Autodesk Fusion 360 part; units mm, degrees
sketch "Sketch1" plane through (0, 0, 0) normal (0, 0, 1) x (1, 0, 0)
  line L0 (4.25, 2.75) -> (-4.25, 2.75)
  line L1 (-4.25, 2.75) -> (-4.25, -2.75)
  line L2 (-4.25, -2.75) -> (4.25, -2.75)
  line L3 (4.25, -2.75) -> (4.25, 2.75)
  line L4 (4.25, 2.75) -> (-4.25, -2.75) construction
  line L5 (-4.25, 2.75) -> (4.25, -2.75) construction
  line L6 (-6.25, -4.75) -> (6.25, -4.75)
  line L7 (6.25, -4.75) -> (6.25, 4.75)
  line L8 (6.25, 4.75) -> (-6.25, 4.75)
  line L9 (-6.25, 4.75) -> (-6.25, -4.75)
  line L10 (-4.25, 2.75) -> (-6.25, 2.75)
  line L11 (4.25, 2.75) -> (6.25, 2.75)
  dimension "d1" = 8.5
  dimension "d2" = 5.5
  dimension "d3" = 2
extrude "Extrude1" add sketch "Sketch1" along normal blind 8.2 contours L1 L2 L3 L6 L7 L9 L10 L11
sketch "Sketch2" plane through (0, 0, 8.2) normal (0, 0, 1) x (-1, 0, 0)
  line L0 (4.25, -2.75) -> (6.25, -2.75)
  line L1 (6.25, -2.75) -> (6.25, 4.75)
  line L2 (6.25, 4.75) -> (-6.25, 4.75)
  line L3 (-6.25, 4.75) -> (-6.25, -2.75)
  line L4 (-6.25, -2.75) -> (-4.25, -2.75)
  line L5 (-4.25, -2.75) -> (-4.25, 2.75)
  line L6 (-4.25, 2.75) -> (4.25, 2.75)
  line L7 (4.25, 2.75) -> (4.25, -2.75)
  line L8 (6.25, -2.75) -> (-6.25, -2.75)
  line L9 (-6.25, -2.75) -> (-6.25, 4.75)
  line L10 (-6.25, 4.75) -> (6.25, 4.75)
  line L11 (6.25, 4.75) -> (6.25, -2.75)
extrude "Extrude2" add sketch "Sketch2" along normal blind 2
sketch "Sketch4" plane through (0, 0, 10.2) normal (0, 0, 1) x (-1, 0, 0)
  line L0 (6.25, 4.75) -> (-6.25, 4.75)
  line L1 (-6.25, 4.75) -> (-6.25, -2.75)
  line L2 (-6.25, -2.75) -> (6.25, -2.75)
  line L3 (6.25, -2.75) -> (6.25, 4.75)
  line L4 (4, -2.75) -> (-4, -2.75)
  line L5 (-4, -2.75) -> (-4, 2.25)
  line L6 (-4, 2.25) -> (4, 2.25)
  line L7 (4, 2.25) -> (4, -2.75)
  line L8 (0, -2.75) -> (0, 4.75) construction
  dimension "d8" = 8
  dimension "d9" = 5
  dimension "d10" = 4
extrude "Extrude3" add sketch "Sketch4" along normal blind 43 contours L2 L4 L5 L6 L7
sketch "Sketch5" plane through (0, -4.75, 0) normal (0, -1, 0) x (1, 0, 0)
  line L0 (-6.25, 0) -> (6.25, 0)
  line L1 (6.25, 0) -> (6.25, 10.2)
  line L2 (6.25, 10.2) -> (-6.25, 10.2)
  line L3 (-6.25, 10.2) -> (-6.25, 0)
  circle A0 centre (0, 3.7) radius 2.15
  line L4 (-4.25, 8.2) -> (4.25, 8.2)
  dimension "d13" = 4.3
  dimension "d18" = 4.5
extrude "Extrude4" cut sketch "Sketch5" against normal blind 2 contours A0
chamfer "Chamfer1" distance 2.2 distance2 5 3 edges at (0, -2.25, 10.2) (4, 0.25, 10.2) (-4, 0.25, 10.2) measured on face at (-1.3333, -3.9167, 10.2) measured on face at (-1.3333, -3.9167, 10.2) measured on face at (-1.3333, -3.9167, 10.2)
extrude "Extrude5" add 1 faces at (-1.4167, -4.0833, 0) along direction (0, 0, -1) blind 0.8
extrude "Extrude6" add 1 faces at (-1.4167, -4.0833, -0.8) along direction (0, 0, -1) blind 5
sketch "Sketch6" plane through (0, 2.75, 0) normal (0, 1, 0) x (-1, 0, 0)
  line L0 (6.25, -5.8) -> (6.25, 10.2)
  line L1 (6.25, 10.2) -> (6.2, 10.2)
  line L2 (6.2, 10.2) -> (4, 15.2)
  line L3 (4, 15.2) -> (4, 53.2)
  line L4 (4, 53.2) -> (-4, 53.2)
  line L5 (-4, 53.2) -> (-4, 15.2)
  line L6 (-4, 15.2) -> (-6.2, 10.2)
  line L7 (-6.2, 10.2) -> (-6.25, 10.2)
  line L8 (-6.25, 10.2) -> (-6.25, -5.8)
  line L9 (-6.25, -5.8) -> (-4.25, -5.8)
  line L10 (-4.25, -5.8) -> (-4.25, 8.2)
  line L11 (-4.25, 8.2) -> (4.25, 8.2)
  line L12 (4.25, 8.2) -> (4.25, -5.8)
  line L13 (4.25, -5.8) -> (6.25, -5.8)
  line L14 (-6.25, -5.8) -> (6.25, -5.8)
  line L15 (6.25, -5.8) -> (6.25, -0.8)
  line L16 (6.25, -0.8) -> (-6.25, -0.8)
  line L17 (-6.25, -0.8) -> (-6.25, -5.8)
  dimension "d23" = 5
  dimension "d28" = 12.5
extrude "Extrude7" add sketch "Sketch6" along normal blind 2 contours L0 L12 L13 L14 L15 L16 | L10 L12 L14 L16 | L8 L9 L10 L14 L16 L17
extrude "Extrude8" cut 1 faces at (1.3333, 1.0833, 53.2) along direction (0, 0, -1) blind 10
equation "d18 = 2.35 mm + 2.15 mm"
Design review of the part built by this model. Coordinates are the model's own, in mm. A direction names the side the tool comes from. Round coordinates to 2 decimals unless told otherwise and drop trailing zeros. Write each loop counter-clockwise with the first axis right and the second up, starting at its lowest first coordinate (ties: lowest second). Pieces come first, ordered by that corner, then holes.
Item 1: Draft analysis for pull direction X (two halves, no side actions). For faces 5 (the flat face through (6.25, -1, 2)), 6 (the flat face through (0, 0, 8.2)), 7 (the flat face through (0, 0, 43.2)), state which applies: released by +X, released by -X, zero draft, split by the parting line, or undercut.
Item 2: Consider section C-C on y = 0. Give the boundary of the cut face in (x, z).
Item 3: Consider section D-D on z = 18. Give the boundary of the cut face in (x, y), and give its area (3 significant figures).
Item 4: Wall thickness on L1, parallel to Z at x = -1, y = -0.25; L2, parallel to Y at x = 3.5, z = 26; L3, parallel to Y at x = -2, z = -1: over which ranges is each line inside the solid? List them lowest first.
Item 5: For faces 1 (the flat face through (0, -2.75, 1)), 2 (the flat face through (0, -2.25, 29)), 3 (the flat face through (-4, 0, 29)), 4 (the flat face through (4, 0, 29)), list the 3-axis set-ups (+Z, -Z, +X, -X, +Y, -Y) from which the entire face can be reached by the end or side of a thin tool; tool diameter is ignored.
Item 6: Consider section B-B on x = 0. Give the boundary of the cut face in (y, z).
Item 7: Consider section A-A on z = 3.7. Give the boundary of the cut face in (x, y).
Item 8: For pin 1 Ø1.5 at (y, z) = (0, 33) entering from +X; pin 2 Ø4 at (x, z) = (-2.5, 31) entering from -Y; pin 3 Ø2.5 at (x, z) = (-2, 4.5) entering from +Y; pin 4 Ø3 at (x, z) = (-1.5, 2.5) entering from -Y, all flat-tipped, find the tip position at first contact; note any pin that passes through.
Check values:
1. face 5: released by +X
1. face 6: undercut
1. face 7: zero draft
2. outline: (-6.25, -5.8) - (-4.25, -5.8) - (-4.25, 8.2) - (4.25, 8.2) - (4.25, -5.8) - (6.25, -5.8) - (6.25, 10.2) - (6.2, 10.2) - (4, 15.2) - (4, 43.2) - (-4, 43.2) - (-4, 15.2) - (-6.2, 10.2) - (-6.25, 10.2) - close
3. outline: (-4, -2.25) - (4, -2.25) - (4, 2.75) - (-4, 2.75) - close
3. area: 40.0 mm2
4. L1: z = 8.2 to 43.2
4. L2: y = -2.25 to 2.75
4. L3: y = -4.75 to -2.75, 2.75 to 4.75
5. face 1: -Z
5. face 2: +Z, +X, -X, -Y
5. face 3: +Z, -X, +Y, -Y
5. face 4: +Z, +X, +Y, -Y
6. outline: (-4.75, -5.8) - (-2.75, -5.8) - (-2.75, 1.55) - (-4.75, 1.55) - close; (-4.75, 5.85) - (-2.75, 5.85) - (-2.75, 8.2) - (2.75, 8.2) - (2.75, 43.2) - (-2.25, 43.2) - (-2.25, 15.2) - (-4.45, 10.2) - (-4.75, 10.2) - close; (2.75, -5.8) - (4.75, -5.8) - (4.75, -0.8) - (2.75, -0.8) - close
7. outline: (-6.25, -4.75) - (-2.15, -4.75) - (-2.15, -2.75) - (-4.25, -2.75) - (-4.25, 2.75) - (-6.25, 2.75) - close; (2.15, -4.75) - (6.25, -4.75) - (6.25, 2.75) - (4.25, 2.75) - (4.25, -2.75) - (2.15, -2.75) - close
8. pin 1: stops at x = 4
8. pin 2: stops at y = -2.25
8. pin 3: stops at y = -2.75
8. pin 4: stops at y = -4.75
